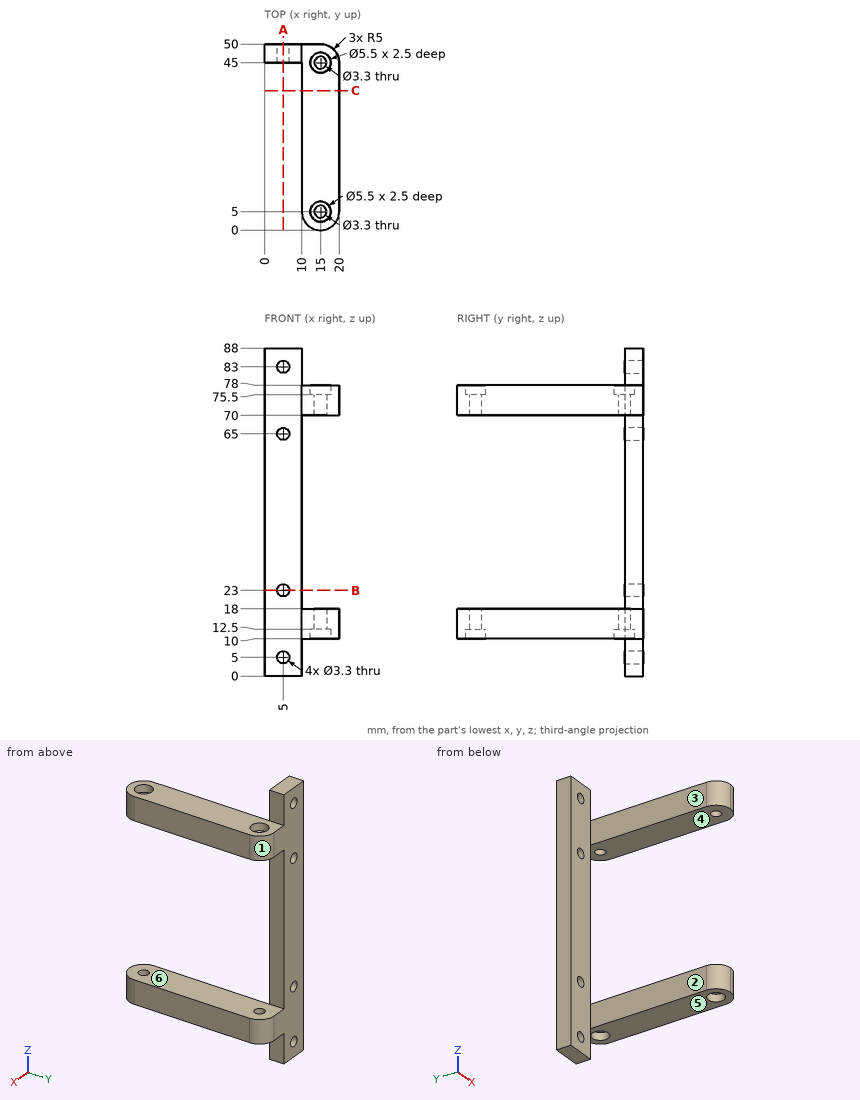
Part print with two shaded views. Sizes in mm from the minimum x, y, z corner. A direction names the side the tool comes from. Give positions to 0.01 mm unless a question says otherwise; leave off trailing zeros. Order: outer loops, then holes, each group sorted by start corner. A loop starts at its lowest first (then second) coordinate and runs counter-clockwise, first axis right, second up.
(1) Saw through at B-B, the plane z = 23. Give the cut face in (x, y).
(2) Drill centre lines: L1, parallel to Z at x = 14, y = 38.5; L2, parallel to X at y = 47, z = 5; L3, parallel to X at y = 9.5, z = 16. Where is each one in solid material? Low to high.
(3) Tool access for the marked faces 1 and 2: list every direction of +Z, -Z, +X, -X, +Y, -Y with a clear straight run to the whole face (end or side of a thin tool).
(4) Mould opens along Z. For the marked faces 3, 4, 5 and 6 say: released by +Z, released by -Z, zero draft, split by the parting line, or undercut.
(5) Saw through at C-C, the plane y = 37.5. Give the cut face in (x, z).
(6) Saw through at A-A, the plane x = 5. Give the cut face in (y, z).
(7) Flat gauge pins, fed straight in: pin 1 (11 mm diameter, centred on x = 16.5, y = 15.5, fed in from -Z); pin 2 (10 mm diameter, centred on y = 35.5, z = 18, fed in from -X); pin 3 (4.5 mm diameter, centred on x = 5, z = 5, fed in from +Y); pin 4 (6.5 mm diameter, centred on x = 15, y = 45, fed in from +Z). Where does each tip first touch, or does it go through?
Results found:
1. outline: (0, 45) - (3.35, 45) - (3.35, 50) - (0, 50) - close; (6.65, 45) - (10, 45) - (10, 50) - (6.65, 50) - close
2. L1: z = 10 to 18, 70 to 78
2. L2: x = 0 to 3.35, 6.65 to 10
2. L3: x = 10 to 20
3. face 1: +Z, -Z, +X, +Y
3. face 2: +Z, -Z, -X, -Y
4. face 3: zero draft
4. face 4: undercut
4. face 5: released by -Z
4. face 6: undercut
5. outline: (10, 10) - (20, 10) - (20, 18) - (10, 18) - close; (10, 70) - (20, 70) - (20, 78) - (10, 78) - close
6. outline: (45, 0) - (50, 0) - (50, 3.35) - (45, 3.35) - close; (45, 6.65) - (50, 6.65) - (50, 21.35) - (45, 21.35) - close; (45, 24.65) - (50, 24.65) - (50, 63.35) - (45, 63.35) - close; (45, 66.65) - (50, 66.65) - (50, 81.35) - (45, 81.35) - close; (45, 84.65) - (50, 84.65) - (50, 88) - (45, 88) - close
7. pin 1: stops at z = 10
7. pin 2: stops at x = 10
7. pin 3: stops at y = 50
7. pin 4: stops at z = 78
